Check sheet for the modelled part. Datum: model origin and axes. Units: mm. A direction names the side the tool comes from. Give positions to 0.01 mm unless a question says otherwise; leave off trailing zeros. Order: outer loops, then holes, each group sorted by start corner. A loop starts at its lowest first (then second) coordinate and runs counter-clockwise, first axis right, second up.
from build123d import *

# Parameters (mm, degrees)
BOSS_EXTRUDE1_DEPTH        = 25.4
SKETCH2_R                  = 4.445
SKETCH2_R_2                = 1.5875
CUT_EXTRUDE1_DEPTH         = 88.683921143
F_10_32_TAPPED_HOLE1_D     = 4.0386
F_10_32_TAPPED_HOLE1_DEPTH = 11.938
F_10_32_TAPPED_HOLE1_TIP   = 1.213317848
FILLET1_R                  = 3.175


with BuildPart() as part:
    # Sketch1 → Boss-Extrude1 (new body)
    with BuildSketch(Plane.XY):
        Polygon((-57.15, -17.035096154), (1.651, -17.035096154), (1.651, 65.514903846), (-4.699, 65.514903846), (-4.699, -7.510096154), (-57.15, -7.510096154), align=None)
    extrude(amount=BOSS_EXTRUDE1_DEPTH)

    # Sketch2 → Cut-Extrude1 (cut, through all)
    with BuildSketch(Plane.ZY.offset(4.699)):
        with Locations(Location((12.7, 50.909903846, 0), (0, 0, 270))):
            Circle(SKETCH2_R)
        with Locations(Location((12.7, 59.863403846, 0), (0, 0, 270))):
            Circle(SKETCH2_R_2)
        with Locations(Location((12.7, 41.956403846, 0), (0, 0, 270))):
            Circle(SKETCH2_R_2)
    extrude(amount=-CUT_EXTRUDE1_DEPTH, mode=Mode.SUBTRACT)

    # #10-32 Tapped Hole1
    with Locations(Plane.ZY.offset(57.15)):
        with Locations((6.985, -12.272596154), (18.415, -12.272596154)):
            Hole(F_10_32_TAPPED_HOLE1_D / 2, depth=F_10_32_TAPPED_HOLE1_DEPTH)
            with Locations((0, 0, -(F_10_32_TAPPED_HOLE1_DEPTH + F_10_32_TAPPED_HOLE1_TIP / 2))):  # 118° drill point
                Cone(0, F_10_32_TAPPED_HOLE1_D / 2, F_10_32_TAPPED_HOLE1_TIP, mode=Mode.SUBTRACT)

    # Fillet1
    fillet1_edges = [part.edges().sort_by_distance(p)[0] for p in [
        (-4.699, -7.510096154, 12.7),
    ]]
    fillet(fillet1_edges, radius=FILLET1_R)


solid = part.part
1) Section check D-D, the plane x = -10. Record the cut outline in (y, z), then the cut area to 3 significant figures.
Recorded:
outline: (-17.04, 0) - (-7.51, 0) - (-7.51, 25.4) - (-17.04, 25.4) - close
area: 242 mm2
2) Material ranges on L1, parallel to Y at x = -43, z = 2.75; L2, parallel to X at y = 12, z = 2; L3, parallel to Y at x = -1, z = 14, recorded low to high.
Recorded:
L1: y = -17.04 to -7.51
L2: x = -4.7 to 1.65
L3: y = -17.04 to 41.05, 42.87 to 46.66, 55.16 to 58.95, 60.77 to 65.51
3) Section check B-B, the plane y = 50.5. Record the cut outline in (x, z).
Recorded:
outline: (-4.7, 0) - (1.65, 0) - (1.65, 8.27) - (-4.7, 8.27) - close; (-4.7, 17.13) - (1.65, 17.13) - (1.65, 25.4) - (-4.7, 25.4) - close
4) Depth check by flat-ended pin: pin 1 Ø10 at (x, z) = (-28, 12.5) entering from +Y; pin 2 Ø5 at (y, z) = (40, 4) entering from -X; pin 3 Ø3.5 at (y, z) = (-12.27, 6.98) entering from -X. Enter the tip coordinate at first touch or a pass-through.
Recorded:
pin 1: stops at y = -7.51
pin 2: stops at x = -4.7
pin 3: stops at x = -45.05
5) Draft check along Y on faces 1 (the face through (-32, -7.51, 13)), 2 (the face through (-1.568, 43.542, 12.77)), 3 (the face through (-28, -17.035, 13)), 4 (the face through (1.651, 24, 13)). Enter one of: +Y half, -Y half, draft (parallel to the pull), parting line (faces both ways), or undercut.
Recorded:
face 1: +Y half
face 2: undercut
face 3: -Y half
face 4: draft
6) Section check A-A, the plane z = 12.7. Record the cut outline in (x, y) (3 decimals).
Recorded:
outline: (-57.15, -17.035) - (1.651, -17.035) - (1.651, 40.369) - (-4.699, 40.369) - (-4.699, -4.335) arc R3.175 cw to (-7.874, -7.51) - (-57.15, -7.51) - close; (-4.699, 43.544) - (1.651, 43.544) - (1.651, 46.465) - (-4.699, 46.465) - close; (-4.699, 55.355) - (1.651, 55.355) - (1.651, 58.276) - (-4.699, 58.276) - close; (-4.699, 61.451) - (1.651, 61.451) - (1.651, 65.515) - (-4.699, 65.515) - close
7) Section check C-C, the plane y = 5. Record the cut outline in (x, z), then the cut area to 3 significant figures.
Recorded:
outline: (-4.7, 0) - (1.65, 0) - (1.65, 25.4) - (-4.7, 25.4) - close
area: 161 mm2
8) Set-up check for faces 5 (the face through (-4.699, 31, 13)), 6 (the face through (-57.15, -12, 13)), 7 (the face through (-51.097, -14.064, 6.053)): record each of +Z, -Z, +X, -X, +Y, -Y from which the full face is reachable in a straight line by a thin tool's end or side.
Recorded:
face 5: +Z, -Z, -X, +Y
face 6: +Z, -Z, -X, +Y, -Y
face 7: -X
